Verification items for this drawing (mm, ordinates from the low corner). A direction names the side the tool comes from. Coordinates: 2 decimals unless noted, no trailing zeros. Write each loop counter-clockwise with the first axis right and the second up, starting at its lowest first coordinate (ties: lowest second). Pieces come first, ordered by that corner, then holes. Notation, with made-up numbers: (80.25, 65.25) -> (132.25, 65.25) arc R25 cw to (132.25, 95.25) -> close; hole circle Ø5 at (-13, -2). An arc over 180 degrees is marked (long way). One line per item, written item: value. Start each with the question number.
1) Sectioned sample at C-C on y = 3.25. Enter the section's corners in (x, z), plus the area to 3 significant figures.
2) Sectioned sample at D-D on x = 1.5. Enter the section's corners in (y, z).
3) Scan lines: line 1 along X through (y, z) = (5, 47) (1 decimal); line 2 along Z through (x, y) = (7.5, 8.5); line 3 along X through (y, z) = (7.5, 43.5). Record each from-to range of solid material in increasing order. Write a range as [from, to].
4) Set-up check for the marked faces 1 and 2: record each of +Z, -Z, +X, -X, +Y, -Y from which the full face is reachable in a straight line by a thin tool's end or side.
5) Gauge pin test, flat ends, axial feed: P1, Ø2, axis at y = 4.5, z = 9.5, coming from the -X side; P2, Ø5, axis at x = 2.5, z = 44.5, coming from the +Y side. Record the tip position at first contact, or that the pin passes through.
6) Sectioned sample at A-A on z = 24.5. Enter the section's corners in (x, y) (3 decimals).
7) Sectioned sample at B-B on x = 6. Enter the section's corners in (y, z), plus the area to 3 significant figures.
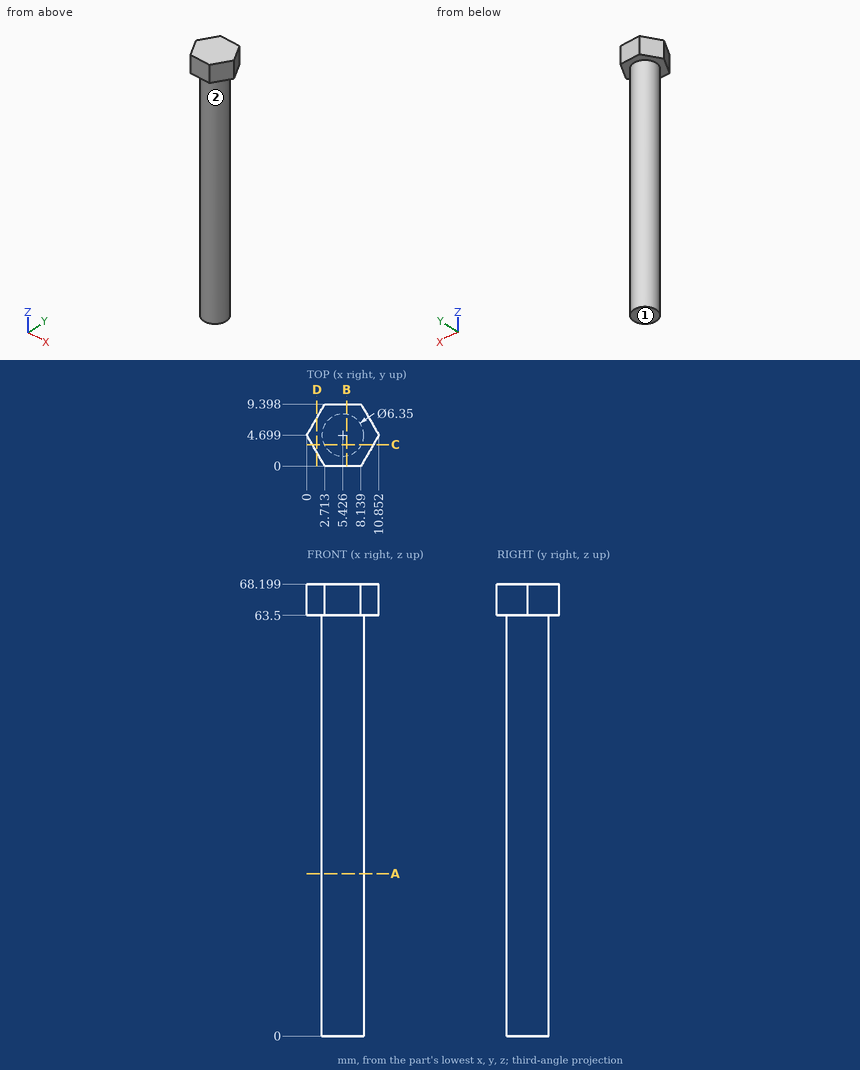
Answers:
1. outline: (0.84, 63.5) -> (2.6, 63.5) -> (2.6, 0) -> (8.25, 0) -> (8.25, 63.5) -> (10.02, 63.5) -> (10.02, 68.2) -> (0.84, 68.2) -> close
1. area: 402 mm2
2. outline: (2.1, 63.5) -> (7.3, 63.5) -> (7.3, 68.2) -> (2.1, 68.2) -> close
3. line 1: x = [2.3, 8.6]
3. line 2: z = [63.5, 68.2]
3. line 3: x = [3.93, 6.92]
4. face 1: -Z, +X, -X, +Y, -Y
4. face 2: -Z
5. P1: stops at x = 2.25
5. P2: stops at y = 7.85
6. outline: circle Ø6.35 at (5.426, 4.699)
7. outline: (0, 63.5) -> (1.58, 63.5) -> (1.58, 0) -> (7.82, 0) -> (7.82, 63.5) -> (9.4, 63.5) -> (9.4, 68.2) -> (0, 68.2) -> close
7. area: 441 mm2
